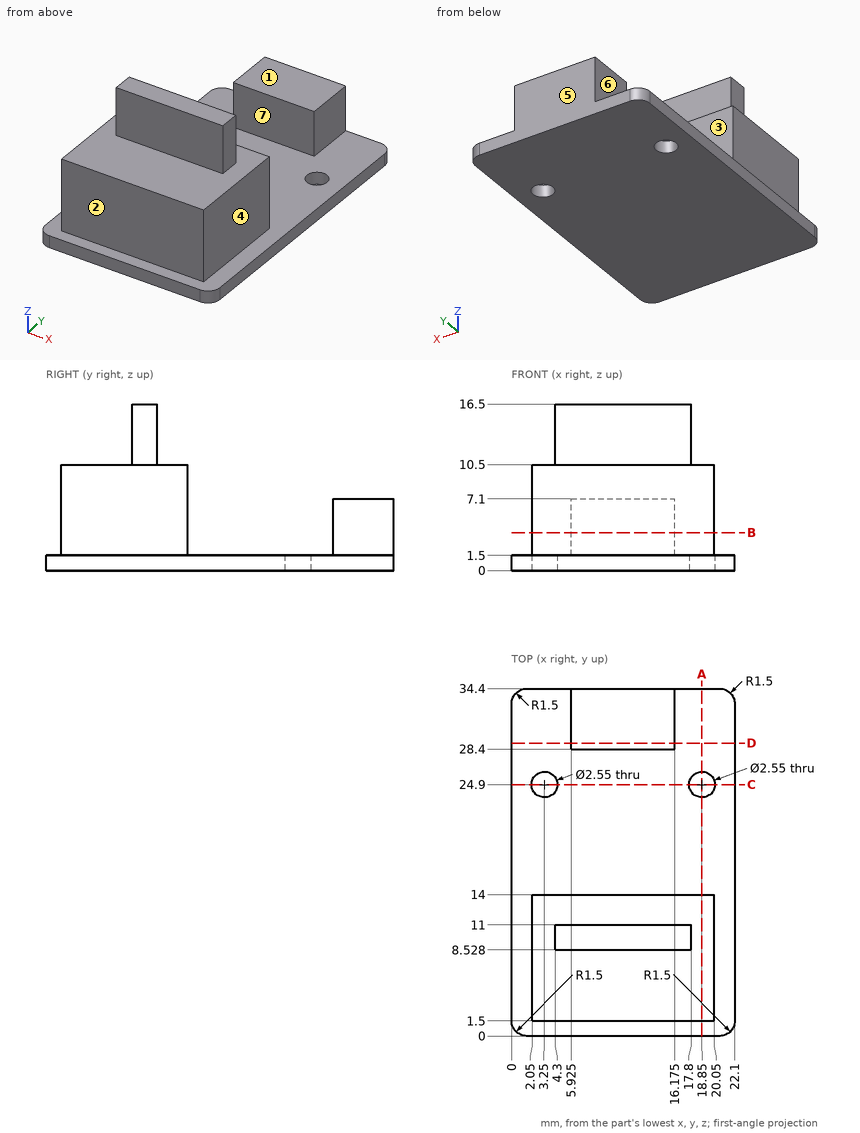
Could you check a few things on this drawing? It's one solid part, dimensions in mm from its lowest x, y, z. A direction names the side the tool comes from. Give positions to 0.01 mm unless a question says otherwise; leave off trailing zeros. Order: outer loops, then holes, each group sorted by start corner. A loop starts at its lowest first (then second) coordinate and runs counter-clockwise, first axis right, second up. Notation, with made-up numbers: (7.25, 65.5) -> (57.25, 65.5) arc R20 cw to (57.25, 70.5) -> close; hole circle Ø2 at (86, 80.25). An arc over 180 degrees is marked (long way). Answer in a Markdown table with one row per item. Add a question column.
Item 1: Imagine slicing it at C-C (y = 24.9). List the corners of the cut face in (x, z) for me (3 decimals), and give its area (3 significant figures).
Item 2: We'd pull the mould along Y, two halves only. Please class the marked faces 5, 6 and 7: pulls with the +Y half, pulls with the -Y half, needs draft (parallel to the pull), parting line crosses it, or undercut.
Item 3: I'm going to push flat-ended pins straight in: P1, Ø3.5, axis at x = 3.25, y = 24.9, coming from the +Z side; P2, Ø1, axis at y = 4, z = 7.5, coming from the +X side; P3, Ø1, axis at x = 17, z = 4.5, coming from the +Y side; P4, Ø10, axis at x = 7, y = 6.5, coming from the +Z side. Where does each tip first touch, or does it pass through?
Item 4: Imagine slicing it at B-B (z = 3.75). List the corners of the cut face in (x, y) for me (3 decimals), and give its area (4 significant figures).
Item 5: Imagine slicing it at D-D (y = 29). List the corners of the cut face in (x, z) for me (3 decimals).
Item 6: Please list where these lines run through material, in increasing order: probe 1 along X at (y, z) = (24.9, 1.15) (1 decimal); probe 2 along Y at (x, z) = (8, 2.25); probe 3 along Y at (x, z) = (18.85, 0.5) (1 decimal).
Item 7: For the marked faces 1, 2, 3 and 4, which set-ups out of +Z, -Z, +X, -X, +Y, -Y let a thin tool reach every point of the face, with its end or its side?
Item 8: Imagine slicing it at A-A (x = 18.85). List the corners of the cut face in (y, z) for me (3 decimals).
Result:
| question | item | result |
|---|---|---|
| 1 | outline | (0, 0) -> (1.975, 0) -> (1.975, 1.5) -> (0, 1.5) -> close; (4.525, 0) -> (17.575, 0) -> (17.575, 1.5) -> (4.525, 1.5) -> close; (20.125, 0) -> (22.1, 0) -> (22.1, 1.5) -> (20.125, 1.5) -> close |
| 1 | area | 25.5 mm2 |
| 2 | face 5 | pulls with the +Y half |
| 2 | face 6 | needs draft |
| 2 | face 7 | undercut |
| 3 | P1 | z = 1.5 |
| 3 | P2 | x = 20.05 |
| 3 | P3 | y = 14 |
| 3 | P4 | z = 16.5 |
| 4 | outline | (2.05, 1.5) -> (20.05, 1.5) -> (20.05, 14) -> (2.05, 14) -> close; (5.925, 28.4) -> (16.175, 28.4) -> (16.175, 34.4) -> (5.925, 34.4) -> close |
| 4 | area | 286.5 mm2 |
| 5 | outline | (0, 0) -> (22.1, 0) -> (22.1, 1.5) -> (16.175, 1.5) -> (16.175, 7.1) -> (5.925, 7.1) -> (5.925, 1.5) -> (0, 1.5) -> close |
| 6 | probe 1 | 0 to 2, 4.5 to 17.6, 20.1 to 22.1 |
| 6 | probe 2 | 1.5 to 14, 28.4 to 34.4 |
| 6 | probe 3 | 0 to 23.6, 26.2 to 34.4 |
| 7 | face 1 | +Z, +X, -X, +Y |
| 7 | face 2 | +Z, +X, -X, -Y |
| 7 | face 3 | +Z, +X, -X |
| 7 | face 4 | +Z, +X, +Y, -Y |
| 8 | outline | (0, 0) -> (23.625, 0) -> (23.625, 1.5) -> (14, 1.5) -> (14, 10.5) -> (1.5, 10.5) -> (1.5, 1.5) -> (0, 1.5) -> close; (26.175, 0) -> (34.4, 0) -> (34.4, 1.5) -> (26.175, 1.5) -> close |
